Geometry check sheet. Reference: the model listing, model coordinates, mm. Face numbers are marked on the shaded views. A direction names the side the tool comes from. Give positions to 0.01 mm unless a question says otherwise; leave off trailing zeros. Loops run counter-clockwise (first coordinate to the right, second up) from the corner with the lowest first, then second, coordinate; pieces in that order, holes last. Notation, with made-up numbers: (-30, 27) -> (-24, 27) arc R15 ccw to (-24, 39) -> close; hole circle Ø7 at (31, 32). An arc over 180 degrees is marked (long way). One line per item, written item: value. Start each with the question number.
(1) Scan lines: line 1 along X through (y, z) = (9, -104.5); line 2 along Y through (x, z) = (-12, -103); line 3 along Y through (x, z) = (4, -49.5). Record each from-to range of solid material in increasing order. Write a range as from..to.
(2) Gauge pin test, flat ends, axial feed: pin 1 Ø9 at (x, z) = (-2, -105.5) entering from +Y; pin 2 Ø6 at (x, z) = (0, 93.5) entering from -Y; pin 3 Ø4 at (x, z) = (0, -104.5) entering from +Y; pin 4 Ø8 at (x, y) = (-6.5, 58) entering from -Z. Record the tip position at first contact, or that the pin passes through.
(3) Sectioned sample at C-C, the plane y = 91.5. Record the cut outline in (x, z).
(4) Sectioned sample at A-A, the plane z = 105.5. Record the cut outline in (x, y).
(5) Tool access check on the marked faces 1, 2 and 3. Record the directions out of +Z, -Z, +X, -X, +Y, -Y that give a thin tool (end or side, any length) a straight path to the whole face; none if there is none.
(6) Sectioned sample at B-B, the plane x = -13.5. Record the cut outline in (y, z), then the cut area to 3 significant figures.
(7) Sectioned sample at D-D, the plane z = 71. Record the cut outline in (x, y), then the cut area to 3 significant figures.
from build123d import *

# Parameters (mm, degrees)
SKETCH1_W               = 40
SKETCH1_H               = 249
BOSS_EXTRUDE1_DEPTH     = 20
SKETCH2_W               = 40
SKETCH2_H               = 40
BOSS_EXTRUDE2_DEPTH     = 89.09
CUT_EXTRUDE1_DEPTH      = 100
CUT_EXTRUDE1_DEPTH_BACK = 10
SKETCH3_W               = 10
SKETCH3_H               = 239
SKETCH6_W               = 30
SKETCH6_H               = 20
CUT_EXTRUDE4_DEPTH      = 20
SKETCH4_R               = 2.35
CUT_EXTRUDE2_DEPTH      = 23
CUT_EXTRUDE3_DEPTH      = 5
SKETCH7_R               = 2.175
CUT_EXTRUDE5_DEPTH      = 8
FILLET1_R               = 3


with BuildPart() as part:
    # Sketch1 → Boss-Extrude1 (new body)
    with BuildSketch(Plane(origin=(0, 0, 0), x_dir=(1, 0, 0), z_dir=(0, 1, 0))):
        Rectangle(SKETCH1_W, SKETCH1_H)
    extrude(amount=BOSS_EXTRUDE1_DEPTH)

    # Sketch2 → Boss-Extrude2 (add)
    with BuildSketch(Plane(origin=(0, 20, 0), x_dir=(1, 0, 0), z_dir=(0, 1, 0))):
        with Locations((0, -104.5)):
            Rectangle(SKETCH2_W, SKETCH2_H)
    extrude(amount=BOSS_EXTRUDE2_DEPTH)

    # Sketch3 → Cut-Extrude1 (cut, two sides: drawn at the far end of the back side and taken through both)
    with BuildSketch(Plane(origin=(0, 20, 0), x_dir=(1, 0, 0), z_dir=(0, 1, 0)).offset(-CUT_EXTRUDE1_DEPTH_BACK)):
        with Locations((-15, 5)):
            Rectangle(SKETCH3_W, SKETCH3_H)
    extrude(amount=CUT_EXTRUDE1_DEPTH + CUT_EXTRUDE1_DEPTH_BACK, mode=Mode.SUBTRACT)

    # Sketch6 → Cut-Extrude4 (cut)
    with BuildSketch(Plane.ZY.offset(10)):
        with Locations((99.5, 30)):
            Rectangle(SKETCH6_W, SKETCH6_H)
    extrude(amount=-CUT_EXTRUDE4_DEPTH, mode=Mode.SUBTRACT)

    # Sketch4 → Cut-Extrude2 (cut)
    with BuildSketch(Plane(origin=(0, 20, 0), x_dir=(1, 0, 0), z_dir=(0, 1, 0))):
        with Locations(Location((0, 104.5, 0), (0, 0, 270))):
            Circle(SKETCH4_R)
        with Locations(Location((0, -105.5, 0), (0, 0, 270))):
            Circle(SKETCH4_R)
    extrude(amount=-CUT_EXTRUDE2_DEPTH, mode=Mode.SUBTRACT)

    # Sketch5 → Cut-Extrude3 (cut)
    with BuildSketch(Plane(origin=(0, 20, 0), x_dir=(1, 0, 0), z_dir=(0, 1, 0))):
        with BuildLine():
            Line((0, 95.5), (-10, 95.5))
            Line((-10, 95.5), (-10, 113.5))
            Line((-10, 113.5), (0, 113.5))
            ThreePointArc((0, 113.5), (9, 104.5), (0, 95.5))
        make_face()
        with BuildLine():
            Line((0, -96.5), (-20, -96.5))
            Line((-20, -96.5), (-20, -114.5))
            Line((-20, -114.5), (0, -114.5))
            ThreePointArc((0, -114.5), (9, -105.5), (0, -96.5))
        make_face()
    extrude(amount=-CUT_EXTRUDE3_DEPTH, mode=Mode.SUBTRACT)

    # Sketch7 → Cut-Extrude5 (cut)
    with BuildSketch(Plane(origin=(20, 0, 0), x_dir=(0, 0, -1), z_dir=(1, 0, 0))):
        with Locations((114.5, 10)):
            Circle(SKETCH7_R)
        with Locations((-115.5, 10)):
            Circle(SKETCH7_R)
        with Locations((-115.5, 99.09)):
            Circle(SKETCH7_R)
    extrude(amount=-CUT_EXTRUDE5_DEPTH, mode=Mode.SUBTRACT)

    # Fillet1
    fillet1_edges = [part.edges().sort_by_distance(p)[0] for p in [
        (20, 109.09, 104.5),
        (0, 0, 124.5),
    ]]
    fillet(fillet1_edges, radius=FILLET1_R)


solid = part.part
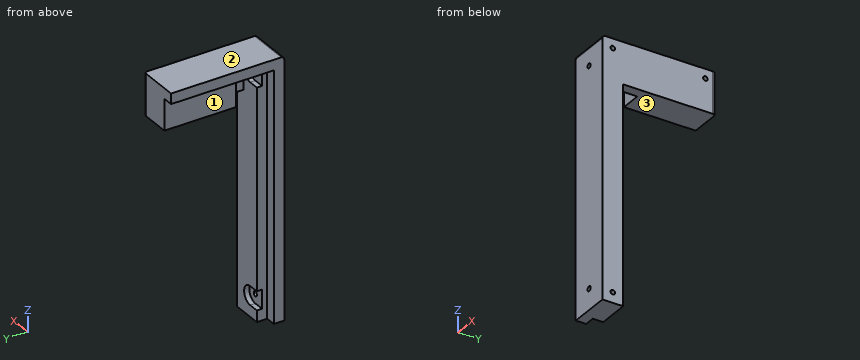
Calculated:
1. line 1: x = -20..-2.35, 2.35..20
1. line 2: y = 0..10
1. line 3: y = 0..20
2. pin 1: stops at y = 15
2. pin 2: stops at y = 0
2. pin 3: passes through
2. pin 4: stops at z = 84.5
3. outline: (-20, 114.5) -> (-10, 114.5) -> (-10, 84.5) -> (20, 84.5) -> (20, 124.5) -> (-20, 124.5) -> close
4. outline: (-20, 0) -> (-2.35, 0) -> (-2.35, 15) -> (-10, 15) -> (-10, 10) -> (-20, 10) -> close; (-10, 40) -> (10, 40) -> (10, 20) -> (9, 20) -> (9, 15) -> (2.35, 15) -> (2.35, 0) -> (20, 0) -> (20, 106.09) arc R3 ccw to (17, 109.09) -> (-10, 109.09) -> close
5. face 1: -Z, -X, +Y
5. face 2: +Z, +X, -X, +Y, -Y
5. face 3: -Z, +X, -X, +Y
6. outline: (0, -124.5) -> (10, -124.5) -> (10, 114.5) -> (109.09, 114.5) -> (109.09, 124.5) -> (3, 124.5) arc R3 ccw to (0, 121.5) -> close
6. area: 3,480 mm2
7. outline: (-20, 0) -> (20, 0) -> (20, 20) -> (-10, 20) -> (-10, 10) -> (-20, 10) -> close
7. area: 700 mm2
